The listing builds one solid part. Answer for the finished solid, in the listing's coordinates (mm). Face numbers are marked on the shaded views. A direction names the side the tool comes from. Round coordinates to 2 decimals unless told otherwise and drop trailing zeros. Answer as a JSON object with one key per item and string values.
```python
from build123d import *

# Parameters (mm, degrees)
SKETCH008_W     = 2.7
SKETCH008_H     = 1.5
PAD_DEPTH       = 20
POCKET_DEPTH    = 5
SKETCH005_R     = 2.917562
POCKET001_DEPTH = 20.6489723154
SKETCH006_R     = 2.917562
POCKET002_DEPTH = 23.0482544438
SKETCH007_R     = 3
POCKET003_DEPTH = 24.3072127265
SKETCH009_R     = 1
POCKET004_DEPTH = 3


with BuildPart() as pad:
    # Sketch008 → Pad (new body, symmetric)
    with BuildSketch(Plane.XZ):
        with Locations((20.330902, 2.75)):
            Rectangle(SKETCH008_W, SKETCH008_H)
        with Locations((-10.535928, 2.75)):
            Rectangle(SKETCH008_W, SKETCH008_H)
        with Locations((-10.535928, 9.489349)):
            Rectangle(SKETCH008_W, SKETCH008_H)
        with Locations((20.330902, 9.48935)):
            Rectangle(SKETCH008_W, SKETCH008_H)
    extrude(amount=PAD_DEPTH, both=True)


with BuildPart() as pocket004:
    # Sketch002 → Loft section 0
    with BuildSketch(Plane.XY.offset(10)):
        with BuildLine():
            ThreePointArc((-11.343506, 11.1193269091), (-20.3555434545, 2.1072894545), (-11.343506, -6.904748))
            Line((-11.343506, -6.904748), (18.7414073452, -6.904748))
            ThreePointArc((18.7414073452, -6.904748), (27.7534447997, 2.1072894545), (18.7414073452, 11.1193269091))
            Line((-11.343506, 11.1193269091), (18.7414073452, 11.1193269091))
        make_face()
    # Sketch003 → Loft section 1
    with BuildSketch(Plane.XY):
        with BuildLine():
            ThreePointArc((-12.0831570349, 16.0971179095), (-26.0729854896, 2.1072894547), (-12.0831570349, -11.882539))
            Line((-12.0831570349, -11.882539), (24.0627546777, -11.882539))
            ThreePointArc((24.0627546777, -11.882539), (38.0525831324, 2.1072894547), (24.0627546777, 16.0971179095))
            Line((-12.0831570349, 16.0971179095), (24.0627546777, 16.0971179095))
        make_face()
    loft()

    # Sketch001 → Pocket (cut)
    with BuildSketch(Plane.XY.offset(10)):
        Polygon((-6.094202, 5.983397), (-6.094202, 8.088668), (11.634386, 7.313041), (14.1254, 6.42784), (13.97268, -0.847062), (13.185631, -1.329644), (-3.545716, -5.318575), (-4.282123, -4.272569), (-6.45014, 0.995308), align=None)
    extrude(amount=-POCKET_DEPTH, mode=Mode.SUBTRACT)

    # Sketch005 → Pocket001 (cut, through all)
    with BuildSketch(Plane(origin=(-6.4881258553, 0.462977012, 0), x_dir=(0.0711766059, 0.9974637291, 0), z_dir=(0.9974637291, -0.0711766059, 0))):
        with Locations((4.141323, 8.428433)):
            Circle(SKETCH005_R)
    extrude(amount=-POCKET001_DEPTH, mode=Mode.SUBTRACT)

    # Sketch006 → Pocket002 (cut, through all)
    with BuildSketch(Plane(origin=(-5.1655859853, -2.1259187014, 0), x_dir=(-0.3805833694, 0.9247466134, 0), z_dir=(0.9247466134, 0.3805833694, 0))):
        with Locations((0.622215, 8.350686)):
            Circle(SKETCH006_R)
    extrude(amount=-POCKET002_DEPTH, mode=Mode.SUBTRACT)

    # Sketch007 → Pocket003 (cut, through all)
    with BuildSketch(Plane(origin=(13.9842993352, -0.2935685174, 0), x_dir=(-0.0209880985, -0.9997797256, 0), z_dir=(-0.9997797256, 0.0209880985, 0))):
        with Locations((-2.85774, 8.49941)):
            Circle(SKETCH007_R)
    extrude(amount=-POCKET003_DEPTH, mode=Mode.SUBTRACT)

    # Cut002: cut Pad
    add(pad.part, mode=Mode.SUBTRACT)

    # Sketch009 → Pocket004 (cut)
    with BuildSketch(Plane(origin=(0, 0, 0), x_dir=(1, 0, 0), z_dir=(0, 0, -1))):
        with Locations((-17.030491, -0.580481)):
            Circle(SKETCH009_R)
        with Locations((28.573694, 1.424915)):
            Circle(SKETCH009_R)
    extrude(amount=-POCKET004_DEPTH, mode=Mode.SUBTRACT)


solid = pocket004.part
```
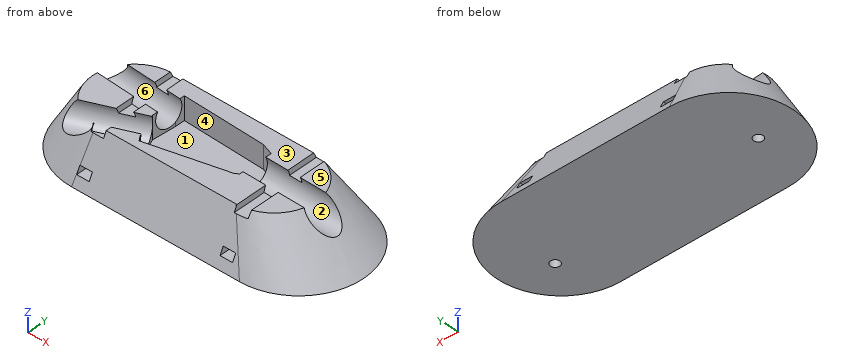
Item 1: Flat-ended cylindrical pins translate along their axes: P1, Ø1, axis at x = 25, z = 7.5, coming from the +Y side; P2, Ø2, axis at x = 27, z = 7.5, coming from the -Y side; P3, Ø1, axis at y = 10.5, z = 9.5, coming from the +X side; P4, Ø3, axis at x = -7, y = 0.5, coming from the -Z side. Find the tip coordinate at first contact, or state that the pin passes through.
Values follow:
{"P1": "y = 11.59", "P2": "y = -6.76", "P3": "x = 24.14", "P4": "z = 0"}
Item 2: Which of the six approach directions +Z, -Z, +X, -X, +Y, -Y give full straight-line access (tool end or side, diameter ignored) to the marked faces 1, 2 and 3?
Values follow:
{"face 1": "+Z", "face 2": "none", "face 3": "+Z, +X, -X, +Y, -Y"}
Item 3: Straight lines are drawn through the part: line 1 (X direction, y = -7.75, z = 2.5); line 2 (Z direction, x = 4.5, y = 3); line 3 (Z direction, x = -7.5, y = -7.25). For each, find the intervals that lie inside material, in ascending order.
Values follow:
{"line 1": "-19.98 to -11.89, -9.19 to 18.98, 21.68 to 30.81", "line 2": "0 to 5", "line 3": "0 to 9.31"}
Item 4: Determine the mould class of the marked faces 4, 5 and 6 for opening direction Y: released by +Y, released by -Y, zero draft, split by the parting line, or undercut.
Values follow:
{"face 4": "undercut", "face 5": "zero draft", "face 6": "undercut"}
Item 5: The part is cut by section A-A (y = 13.25). Give the number of separate pieces and of enclosed holes in the cut face, then the cut area to 3 significant figures.
Values follow:
{"separate pieces": "1", "enclosed holes": "2", "area": "252 mm^2"}
